Source: CAD feature listing. Evaluate the final solid. Frame: model axes, mm. Give positions to 0.01 mm unless a question says otherwise; leave off trailing zeros. Loops run counter-clockwise (first coordinate to the right, second up) from the corner with the lowest first, then second, coordinate; pieces in that order, holes last. Notation, with made-up numbers: (33.5, 67) -> (46.5, 67) arc R19 cw to (46.5, 87) -> close; hole circle Ø8 at (12, 78). An arc over 180 degrees is marked (long way). Return JSON: item names as keys, results as strings. Group by question number.
```python
from build123d import *

# Parameters (mm, degrees)
SKETCH_1_R          = 13
SKETCH_1_R_2        = 11
EXTRUDE_1_DEPTH     = 460
SKETCH_4_R          = 1.5
CUT_EXTRUDE_2_DEPTH = 14
SKETCH_6_R          = 3
CUT_EXTRUDE_3_DEPTH = 14.0000001


with BuildPart() as part:
    # 草图1 → 凸台-拉伸1 (new body)
    with BuildSketch(Plane(origin=(0, 0, 0), x_dir=(0, 0, -1), z_dir=(1, 0, 0))):
        Circle(SKETCH_1_R)
        Circle(SKETCH_1_R_2, mode=Mode.SUBTRACT)
    extrude(amount=EXTRUDE_1_DEPTH)

    # 草图4 → 切除-拉伸2 (cut, through all)
    with BuildSketch(Plane(origin=(0, 0, 0), x_dir=(1, 0, 0), z_dir=(0, 1, 0))):
        with Locations((12.5, 0)):
            Circle(SKETCH_4_R)
        with Locations((441.5, 0)):
            Circle(SKETCH_4_R)
    extrude(amount=-CUT_EXTRUDE_2_DEPTH, mode=Mode.SUBTRACT)

    # 草图6 → 切除-拉伸3 (cut, through all)
    with BuildSketch(Plane.XY):
        with Locations((12.5, 0)):
            Circle(SKETCH_6_R)
    extrude(amount=CUT_EXTRUDE_3_DEPTH, mode=Mode.SUBTRACT)


solid = part.part
```
1) Material intervals for line 1 (X direction, y = -12.3, z = 0); line 2 (Y direction, x = 258, z = 0.5); line 3 (Z direction, x = 79, y = -7.5), sorted ascending.
2) Mould query, pull axis Z, two halves, no side actions, for faces 1 (the face through (226.78, -10.74, 2.38)), 2 (the face through (0, 3, 11)), 3 (the face through (226.78, -7.91, 10.316)). Classes: released by +Z, released by -Z, zero draft, split by the parting line, or undercut.
3) Cut plane B-B on x = 96. Return loops of the section in (y, z).
4) Cut plane A-A on z = -7.25. Return loops of the section in (x, y).
5) Contact query for flat-ended pins moving along their axis: P1, Ø7, axis at x = 12.5, y = 0, coming from the +Z side; P2, Ø1.5, axis at x = 102.5, z = 5, coming from the +Y side; P3, Ø2.5, axis at x = 12.5, z = 0, coming from the -Y side; P4, Ø8, axis at x = 53.5, z = -4.5, coming from the +Y side. Output: stop coordinate, or through.
Calculated:
{
 "1": {"line 1": "0 to 11, 14 to 440, 443 to 460", "line 2": "-12.99 to -10.99, 10.99 to 12.99", "line 3": "-10.62 to -8.05, 8.05 to 10.62"},
 "2": {"face 1": "undercut", "face 2": "zero draft", "face 3": "split by the parting line"},
 "3": {"outline": "circle Ø26 at (0, 0); hole circle Ø22 at (0, 0)"},
 "4": {"outline": "(0, -10.79) -> (460, -10.79) -> (460, -8.27) -> (0, -8.27) -> close; (0, 8.27) -> (460, 8.27) -> (460, 10.79) -> (0, 10.79) -> close"},
 "5": {"P1": "z = 13", "P2": "y = 12.29", "P3": "y = 10.93", "P4": "y = 12.99"}
}
